from build123d import *

# Parameters (mm, degrees)
F0_R     = 3.175
F1_DEPTH = 5.08


# Not quite as in the source:
# - a feature names something its author has since deleted; it is built from what else it names


with BuildPart() as f1:
    # F0 (on Top) → F1 (new body)
    with BuildSketch(Plane.XY):
        Polygon((-196.7800016522, 116.4700038791), (-196.7814051471, 116.4700038791), (-202.7097940445, 116.4700038791), (-202.7097940445, 108.8500038791), (-202.7097940445, 101.2300038791), (-202.7097940445, -23.2299961209), (-196.7800016522, -23.2299961209), (20.8102059555, -23.2299961209), (20.8102059555, 116.4700038791), (15.3085948529, 116.4700038791), (-35.4914051471, 116.4700038791), (-39.3014051471, 116.4700038791), (-90.9497940445, 116.4700038791), (-187.4697940445, 116.4700038791), (-189.1614051471, 116.4700038791), (-195.0897940445, 116.4700038791), align=None)
        with Locations((-196.3344303894, -15.6099961209)):
            Circle(F0_R, mode=Mode.SUBTRACT)
        Polygon((-189.1614051471, -18.3182691255), (-189.1614051471, 111.2217308745), (-189.1583133745, 111.2217308745), (-39.3014051471, 111.2217308745), (-39.3014051471, -18.3182691255), align=None, mode=Mode.SUBTRACT)
        with Locations((14.4348423004, -15.6099961209)):
            Circle(F0_R, mode=Mode.SUBTRACT)
        Polygon((0, 52.8017308745), (0, 46.4517308745), (0, 40.1017308745), (-6.35, 40.1017308745), (-6.35, 46.4517308745), (-6.35, 52.8017308745), align=None, mode=Mode.SUBTRACT)
        with Locations((-196.3344303894, 108.8500038791)):
            Circle(F0_R, mode=Mode.SUBTRACT)
        with Locations((14.4348423004, 108.8500038791)):
            Circle(F0_R, mode=Mode.SUBTRACT)
    extrude(amount=F1_DEPTH)


solid = f1.part
Work out the finished part from the listing and answer in its coordinate system (mm). A direction names the side the tool comes from. Coordinates: 2 decimals unless noted, no trailing zeros. Loops run counter-clockwise (first coordinate to the right, second up) from the corner with the lowest first, then second, coordinate; pieces in that order, holes last. Notation, with made-up numbers: M -7.75,-18 L 38.25,-18 A22 ccw 38.25,11 Z; hole C -25,80.5 d4. An arc over 180 degrees is marked long. Answer in a Markdown table with one row per item. Add a question column.
1. Find section B-B, the plane y = 65. Write down the section's boundary in (x, z), then the cut area to 3 significant figures.
2. Consider L1, parallel to X at y = 45, z = 4.4; L2, parallel to X at y = 81, z = 3.3; L3, parallel to Y at x = -89, z = 3.1. Determine where each line is inside the solid, lowest interval first.
3. Find section A-A, the plane x = -140. Write down the section's boundary in (y, z), then the cut area to 3 significant figures.
4. The mould has two halves that part along Y. Classify faces 1 (the flat face through (-3, 52.802, 3)), 2 (the flat face through (-93, -23.23, 3)), 3 (the flat face through (-202.71, 48, 3)): pulls with the +Y half, pulls with the -Y half, needs draft (parallel to the pull), parting line crosses it, or undercut.
5. Find section C-C, the plane z = 2.95. Write down the section's boundary in (x, y) (3 decimals), then the cut area to 3 significant figures.
6. A tool of negligible diameter and unlimited length cuts with its end or side. For faces 4 (the flat face through (-6.35, 46, 3)), 5 (the flat face through (-34, 42, 5.08)), from which of +Z, -Z, +X, -X, +Y, -Y can it reach the whole face along a straight path? Write none if from no direction.
Reported:
| question | item | result |
|---|---|---|
| 1 | outline | M -202.71,0 L -189.16,0 L -189.16,5.08 L -202.71,5.08 Z; M -39.3,0 L 20.81,0 L 20.81,5.08 L -39.3,5.08 Z |
| 1 | area | 374 mm^2 |
| 2 | L1 | x = -202.71 to -189.16, -39.3 to -6.35, 0 to 20.81 |
| 2 | L2 | x = -202.71 to -189.16, -39.3 to 20.81 |
| 2 | L3 | y = -23.23 to -18.32, 111.22 to 116.47 |
| 3 | outline | M -23.23,0 L -18.32,0 L -18.32,5.08 L -23.23,5.08 Z; M 111.22,0 L 116.47,0 L 116.47,5.08 L 111.22,5.08 Z |
| 3 | area | 51.6 mm^2 |
| 4 | face 1 | undercut |
| 4 | face 2 | pulls with the -Y half |
| 4 | face 3 | needs draft |
| 5 | outline | M -202.71,-23.23 L 20.81,-23.23 L 20.81,116.47 L -202.71,116.47 Z; hole C -196.334,-15.61 d6.35; hole C -196.334,108.85 d6.35; hole M -189.161,-18.318 L -39.301,-18.318 L -39.301,111.222 L -189.161,111.222 Z; hole M -6.35,40.102 L 0,40.102 L 0,52.802 L -6.35,52.802 Z; hole C 14.435,-15.61 d6.35; hole C 14.435,108.85 d6.35 |
| 5 | area | 11,600 mm^2 |
| 6 | face 4 | +Z, -Z |
| 6 | face 5 | +Z, +X, -X, +Y, -Y |
